Build history of the part. All positions in model axes, mm. Face numbers are marked on the shaded views. Coordinates: 2 decimals unless noted, no trailing zeros. Write each loop counter-clockwise with the first axis right and the second up, starting at its lowest first coordinate (ties: lowest second). Pieces come first, ordered by that corner, then holes.
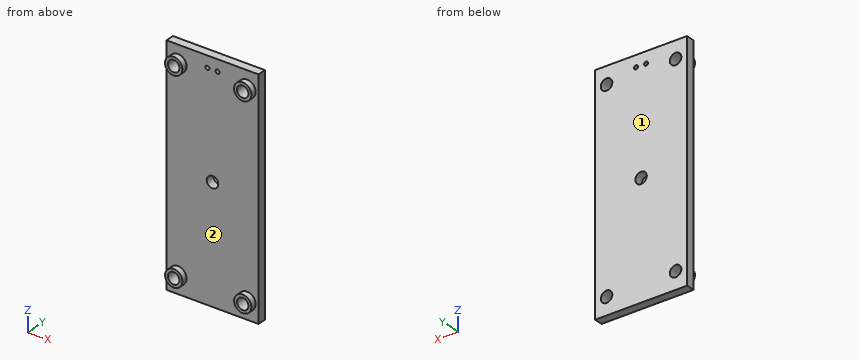
from build123d import *

# Parameters (mm, degrees)
SKETCH1_W           = 203.2
SKETCH1_H           = 508
BASE_EXTRUDE_DEPTH  = 19.05
SKETCH2_R           = 19.05
BOSS_EXTRUDE1_DEPTH = 12.7
SKETCH3_R           = 12.7
CUT_EXTRUDE1_DEPTH  = 520.032390608
SKETCH4_R           = 12.7
CUT_EXTRUDE2_DEPTH  = 520.032390608
SKETCH5_R           = 4.365625
CUT_EXTRUDE3_DEPTH  = 519.410515422


with BuildPart() as part:
    # Sketch1 → Base-Extrude (new body)
    with BuildSketch(Plane(origin=(0, 0, 0), x_dir=(1, 0, 0), z_dir=(0, 1, 0))):
        with Locations((0, -254)):
            Rectangle(SKETCH1_W, SKETCH1_H)
    extrude(amount=BASE_EXTRUDE_DEPTH)

    # Sketch2 → Boss-Extrude1 (add)
    with BuildSketch(Plane.XZ):
        with Locations(Location((76.2, 469.9, 0), (0, 0, 270))):
            Circle(SKETCH2_R)
        with Locations(Location((76.2, 38.1, 0), (0, 0, 90))):
            Circle(SKETCH2_R)
        with Locations(Location((-76.2, 38.1, 0), (0, 0, 270))):
            Circle(SKETCH2_R)
        with Locations(Location((-76.2, 469.9, 0), (0, 0, 90))):
            Circle(SKETCH2_R)
    extrude(amount=BOSS_EXTRUDE1_DEPTH)

    # Sketch3 → Cut-Extrude1 (cut, through all)
    with BuildSketch(Plane.XZ.offset(12.7)):
        with Locations(Location((76.2, 469.9, 0), (0, 0, 270))):
            Circle(SKETCH3_R)
        with Locations(Location((-76.2, 469.9, 0), (0, 0, 270))):
            Circle(SKETCH3_R)
        with Locations(Location((76.2, 38.1, 0), (0, 0, 270))):
            Circle(SKETCH3_R)
        with Locations(Location((-76.2, 38.1, 0), (0, 0, 270))):
            Circle(SKETCH3_R)
    extrude(amount=-CUT_EXTRUDE1_DEPTH, mode=Mode.SUBTRACT)

    # Sketch4 → Cut-Extrude2 (cut, through all)
    with BuildSketch(Plane(origin=(0, 19.05, 0), x_dir=(-1, 0, 0), z_dir=(0, 1, 0))):
        with Locations(Location((0, 254, 0), (0, 0, 90))):
            Circle(SKETCH4_R)
    extrude(amount=-CUT_EXTRUDE2_DEPTH, mode=Mode.SUBTRACT)

    # Sketch5 → Cut-Extrude3 (cut, through all)
    with BuildSketch(Plane.XZ):
        with Locations(Location((11.1125, 482.6, 0), (0, 0, 270))):
            Circle(SKETCH5_R)
        with Locations(Location((-11.1125, 482.6, 0), (0, 0, 270))):
            Circle(SKETCH5_R)
    extrude(amount=-CUT_EXTRUDE3_DEPTH, mode=Mode.SUBTRACT)


solid = part.part
(1) Slice it at C-C, the plane z = 469.9. List the corners of the cut face in (x, y).
(2) Two-plate mould, pull along Z, no slides. Class the marked faces 1 and 2: pulls with the +Z half, pulls with the -Z half, needs draft (parallel to the pull), parting line crosses it, or undercut.
(3) Probe L1, parallel to Z at x = -76, y = 7; L2, parallel to Z at x = 1.5, y = 16.5; L3, parallel to X at y = 14.5, z = 254. List the from-to ranges inside material, lowest first.
(4) Slice it at A-A, the plane x = 76.2. List the corners of the cut face in (y, z).
(5) Slice it at B-B, the plane z = 254. List the corners of the cut face in (x, y), and give its area (3 significant figures).
(6) Flat gauge pin, fed straight in: P1, Ø6, axis at x = 25, z = 343, coming from the -Y side. Where does the tip first touch, or does it go through?
(7) Slice it at D-D, the plane x = 0. List the corners of the cut face in (y, z).
Results:
1. outline: (-101.6, 0) - (-95.25, 0) - (-95.25, -12.7) - (-88.9, -12.7) - (-88.9, 19.05) - (-101.6, 19.05) - close; (-63.5, -12.7) - (-57.15, -12.7) - (-57.15, 0) - (57.15, 0) - (57.15, -12.7) - (63.5, -12.7) - (63.5, 19.05) - (-63.5, 19.05) - close; (88.9, -12.7) - (95.25, -12.7) - (95.25, 0) - (101.6, 0) - (101.6, 19.05) - (88.9, 19.05) - close
2. face 1: needs draft
2. face 2: undercut
3. L1: z = 0 to 25.4, 50.8 to 457.2, 482.6 to 508
3. L2: z = 0 to 241.39, 266.61 to 508
3. L3: x = -101.6 to -12.7, 12.7 to 101.6
4. outline: (-12.7, 19.05) - (0, 19.05) - (0, 0) - (19.05, 0) - (19.05, 25.4) - (-12.7, 25.4) - close; (-12.7, 50.8) - (19.05, 50.8) - (19.05, 457.2) - (-12.7, 457.2) - (-12.7, 450.85) - (0, 450.85) - (0, 57.15) - (-12.7, 57.15) - close; (-12.7, 482.6) - (19.05, 482.6) - (19.05, 508) - (0, 508) - (0, 488.95) - (-12.7, 488.95) - close
5. outline: (-101.6, 0) - (-12.7, 0) - (-12.7, 19.05) - (-101.6, 19.05) - close; (12.7, 0) - (101.6, 0) - (101.6, 19.05) - (12.7, 19.05) - close
5. area: 3,390 mm2
6. P1: stops at y = 0
7. outline: (0, 0) - (19.05, 0) - (19.05, 241.3) - (0, 241.3) - close; (0, 266.7) - (19.05, 266.7) - (19.05, 508) - (0, 508) - close
